```python
from build123d import *

# Parameters (mm, degrees)
SALIENTE_EXTRUIR1_DEPTH      = 16
SALIENTE_EXTRUIR1_DEPTH_BACK = 16
CORTAR_EXTRUIR1_DEPTH        = 49.25
CORTAR_EXTRUIR1_DEPTH_BACK   = 49.25
CROQUIS3_R                   = 4.8
CORTAR_EXTRUIR2_DEPTH        = 25.3
CROQUIS4_R                   = 4.8
CORTAR_EXTRUIR3_DEPTH        = 25.3
CROQUIS6_W                   = 64
CROQUIS6_H                   = 50.5
CORTAR_EXTRUIR4_DEPTH        = 98.5
CORTAR_EXTRUIR4_DEPTH_BACK   = 98.5
CROQUIS7_W                   = 118.5
CROQUIS7_H                   = 52
CORTAR_EXTRUIR5_DEPTH        = 25.3


with BuildPart() as part:
    # Croquis1 → Saliente-Extruir1 (new body, two sides)
    with BuildSketch(Plane.XY) as saliente_extruir1_sk:
        with BuildLine():
            Line((-49.25, -23.8), (-49.25, -25.3))
            Line((-49.25, -25.3), (-29.12605042, -25.3))
            ThreePointArc((-29.12605042, -25.3), (-26.427107301, -24.400792418), (-24.806790899, -22.062536016))
            Line((-24.806790899, -22.062536016), (-23.194455177, -16.5465774))
            ThreePointArc((-23.194455177, -16.5465774), (-21.665135808, -15.146167956), (-19.716192024, -15.854392832))
            ThreePointArc((-19.716192024, -15.854392832), (0, -25.3), (19.716192024, -15.854392832))
            ThreePointArc((19.716192024, -15.854392832), (21.665135808, -15.146167956), (23.194455177, -16.5465774))
            Line((23.194455177, -16.5465774), (24.806790899, -22.062536016))
            ThreePointArc((24.806790899, -22.062536016), (26.427107301, -24.400792418), (29.12605042, -25.3))
            Line((29.12605042, -25.3), (49.25, -25.3))
            Line((49.25, -25.3), (49.25, -23.8))
            Line((49.25, -23.8), (29.12605042, -23.8))
            ThreePointArc((29.12605042, -23.8), (27.326755007, -23.200528279), (26.246544073, -21.641690678))
            Line((26.246544073, -21.641690678), (22.185653478, -7.748985725))
            ThreePointArc((22.185653478, -7.748985725), (0, -23.5), (-22.185653478, -7.748985725))
            Line((-22.185653478, -7.748985725), (-26.246544073, -21.641690678))
            ThreePointArc((-26.246544073, -21.641690678), (-27.326755007, -23.200528279), (-29.12605042, -23.8))
            Line((-29.12605042, -23.8), (-49.25, -23.8))
        make_face()
    extrude(amount=SALIENTE_EXTRUIR1_DEPTH)
    extrude(saliente_extruir1_sk.sketch, amount=-SALIENTE_EXTRUIR1_DEPTH_BACK)

    # Croquis2 → Cortar-Extruir1 (cut, two sides)
    with BuildSketch(Plane(origin=(0, 0, 0), x_dir=(0, 0, -1), z_dir=(1, 0, 0))) as cortar_extruir1_sk:
        Polygon((-16, -25.3), (-10.5, 0), (-10.5, 25.2), (10.5, 25.2), (10.5, 0), (16, -25.3), (16, 26.2), (-16, 26.2), align=None)
    extrude(amount=CORTAR_EXTRUIR1_DEPTH, mode=Mode.SUBTRACT)
    extrude(cortar_extruir1_sk.sketch, amount=-CORTAR_EXTRUIR1_DEPTH_BACK, mode=Mode.SUBTRACT)

    # Croquis3 → Cortar-Extruir2 (cut)
    with BuildSketch(Plane(origin=(0, 0, 0), x_dir=(1, 0, 0), z_dir=(0, 1, 0))):
        with Locations((38, 0)):
            Circle(CROQUIS3_R)
    extrude(amount=-CORTAR_EXTRUIR2_DEPTH, mode=Mode.SUBTRACT)

    # Croquis4 → Cortar-Extruir3 (cut)
    with BuildSketch(Plane(origin=(0, 0, 0), x_dir=(1, 0, 0), z_dir=(0, 1, 0))):
        with Locations((-38, 0)):
            Circle(CROQUIS4_R)
    extrude(amount=-CORTAR_EXTRUIR3_DEPTH, mode=Mode.SUBTRACT)

    # Croquis5 → Revoluci_n1 (revolve)
    with BuildSketch(Plane(origin=(0, 0, 0), x_dir=(0, 0, -1), z_dir=(1, 0, 0))):
        with BuildLine():
            Line((-10.5, -19.709677419), (-10.5, -23.65))
            Line((-10.5, -23.65), (10.5, -23.65))
            Line((10.5, -23.65), (10.5, -19.709677419))
            Line((10.5, -19.709677419), (8.8, -19.709677419))
            Line((8.8, -19.709677419), (8.60641193, -21.293920434))
            ThreePointArc((8.60641193, -21.293920434), (8.395381567, -21.796423837), (7.952186088, -22.113632366))
            ThreePointArc((7.952186088, -22.113632366), (-4.5e-08, -23.5), (-7.952186172, -22.113632336))
            ThreePointArc((-7.952186172, -22.113632336), (-8.395381595, -21.796423802), (-8.60641193, -21.293920434))
            Line((-8.60641193, -21.293920434), (-8.8, -19.709677419))
            Line((-8.8, -19.709677419), (-10.5, -19.709677419))
        make_face()
    revolve(axis=Axis((0, 0, 16), (0, 0, -1)))

    # Croquis6 → Cortar-Extruir4 (cut, two sides)
    with BuildSketch(Plane(origin=(0, 0, 0), x_dir=(0, 0, -1), z_dir=(1, 0, 0))) as cortar_extruir4_sk:
        with Locations((0, 11.1)):
            Rectangle(CROQUIS6_W, CROQUIS6_H)
    extrude(amount=CORTAR_EXTRUIR4_DEPTH, mode=Mode.SUBTRACT)
    extrude(cortar_extruir4_sk.sketch, amount=-CORTAR_EXTRUIR4_DEPTH_BACK, mode=Mode.SUBTRACT)

    # Croquis7 → Cortar-Extruir5 (cut)
    with BuildSketch(Plane(origin=(0, 0, 0), x_dir=(1, 0, 0), z_dir=(0, 1, 0))):
        Rectangle(CROQUIS7_W, CROQUIS7_H)
        Polygon((-49.25, 16), (-49.25, -16), (-34.16469212, -16), (-30.107815494, -7.3), (-19.2, -7.3), (-16, -10.5), (16, -10.5), (19.2, -7.3), (30.107815494, -7.3), (34.16469212, -16), (49.25, -16), (49.25, 16), (34.16469212, 16), (30.107815494, 7.3), (19.2, 7.3), (16, 10.5), (-16, 10.5), (-19.2, 7.3), (-30.107815494, 7.3), (-34.16469212, 16), align=None, mode=Mode.SUBTRACT)
    extrude(amount=-CORTAR_EXTRUIR5_DEPTH, mode=Mode.SUBTRACT)


solid = part.part
```
Can you work these out from the model? Positions are in its coordinate system, mm. A direction names the side the tool comes from. Coordinates: 2 decimals unless noted, no trailing zeros. Order: outer loops, then holes, each group sorted by start corner. A loop starts at its lowest first (then second) coordinate and runs counter-clockwise, first axis right, second up.
1. For faces 5 (the face through (-25, -20, 7.3)), 6 (the face through (25, -20, -7.3)), 7 (the face through (24, -19.3, 0.1)), 8 (the face through (0.24, -19.96, 8.77)), which set-ups out of +Z, -Z, +X, -X, +Y, -Y let a thin tool reach every point of the face, with its end or its side?
2. If we section it at B-B (z = -12.5): Please give me the cut outline in (x, y).
3. Thinking about a two-plate mould opening in Z: for faces 1 (the face through (-33.42, -24.54, -1.44)), 2 (the face through (25, -19, 7.3)), 3 (the face through (32.165, -24.54, -11.711)), 4 (the face through (27.35, -23.22, 0.1)), which applies, +Z half, -Z half, draft (parallel to the pull), parting line (faces both ways), or undercut?
4. I'm going to push flat-ended pins straight in: pin 1 (3.5 mm diameter, centred on x = 8, y = -22.5, fed in from -Z); pin 2 (3.5 mm diameter, centred on x = 23.5, y = -22, fed in from +Z); pin 3 (10 mm diameter, centred on x = 42.5, z = -5, fed in from +Y). Where does each tip first touch, or does it pass through?
5. I need wall thicknesses on line 1 (X direction, y = -18.75, z = -2); line 2 (X direction, y = -21, z = -3); line 3 (Y direction, x = -35.5, z = -9). Which ranges of each line are inside material? Lowest first, please.
6. If we section it at A-A (x = 38): Please give me the cut outline in (y, z), then the cut area to 3 significant figures.
Entries:
1. face 5: +Z, +Y, -Y
1. face 6: -Z, +Y, -Y
1. face 7: +Z, -Z, -Y
1. face 8: +Y
2. outline: (-49.25, -25.3) - (-32.53, -25.3) - (-32.53, -23.8) - (-49.25, -23.8) - close; (32.53, -25.3) - (49.25, -25.3) - (49.25, -23.8) - (32.53, -23.8) - close
3. face 1: undercut
3. face 2: +Z half
3. face 3: -Z half
3. face 4: draft
4. pin 1: stops at z = -10.5
4. pin 2: stops at z = 7.3
4. pin 3: stops at y = -23.8
5. line 1: x = -25.4 to -23.84, -16.99 to -14.02, 14.02 to 16.99, 23.84 to 25.4
5. line 2: x = -26.06 to -24.5, -14.11 to -10.11, 10.11 to 14.11, 24.5 to 26.06
5. line 3: y = -25.3 to -23.8
6. outline: (-25.3, -16) - (-23.8, -15.67) - (-23.8, -4.8) - (-25.3, -4.8) - close; (-25.3, 4.8) - (-23.8, 4.8) - (-23.8, 15.67) - (-25.3, 16) - close
6. area: 33.1 mm2
